Read the model definition and answer for the solid it produces. Units are mm, in the model's axes. A direction names the side the tool comes from. Give positions to 0.01 mm unless a question says otherwise; leave off trailing zeros. Write each loop counter-clockwise with the first axis right and the second up, starting at its lowest first coordinate (ties: lowest second). Pieces come first, ordered by that corner, then holes. Notation, with made-up numbers: M 53.25,58 L 80.25,58 A6 cw 80.25,68 Z; hole C 48,67 d7. An arc over 180 degrees is marked long. Put each result on its own line as item: value.
Autodesk Inventor part; units mm, degrees
ref_plane "YZ Plane" through (0, 0, 0) normal (1, 0, 0) x (0, 1, 0)
ref_plane "XZ Plane" through (0, 0, 0) normal (0, 1, 0) x (-1, 0, 0)
ref_plane "XY Plane" through (0, 0, 0) normal (0, 0, 1) x (1, 0, 0)
sketch "Sketch1" plane through (0, 0, 0) normal (0, 1, 0) x (-1, 0, 0)
  line L0 (0, 0) -> (-25, 0)
  line L1 (-25, 0) -> (-25, 25)
  line L2 (-25, 25) -> (0, 25)
  line L3 (0, 25) -> (0, 0)
  circle A0 centre (-4.5, 4.5) radius 4
  circle A1 centre (-4.5, 20.5) radius 4
  circle A2 centre (-20.5, 20.5) radius 4
  circle A3 centre (-20.5, 4.5) radius 4
  dimension "d0" = 25
  dimension "d1" = 25
  dimension "d2" = 8
  dimension "d3" = 8
  dimension "d4" = 8
  dimension "d5" = 8
extrude "Extrusion1" add sketch "Sketch1" along normal blind 5
sketch "Sketch2" plane through (0, 5, 0) normal (0, 1, 0) x (1, 0, 0)
  line L0 (0, 0) -> (0, -25)
  line L1 (25, -25) -> (25, 0)
  line L2 (0, -25) -> (25, -25)
  line L3 (25, -25) -> (25, 0)
  line L4 (25, 0) -> (0, 0)
  line L5 (0, 0) -> (0, -25)
extrude "Extrusion2" add sketch "Sketch2" along normal blind 5
sketch "Sketch4" plane through (0, 0, 0) normal (0, -1, 0) x (1, 0, 0)
  line L0 (9.5, 3) -> (15.5, 3)
  line L1 (15.5, 3) -> (15.5, 6)
  line L2 (15.5, 6) -> (9.5, 6)
  line L3 (9.5, 6) -> (9.5, 3)
  line L4 (9.5, 22) -> (15.5, 22)
  line L5 (15.5, 22) -> (15.5, 19)
  line L6 (15.5, 19) -> (9.5, 19)
  line L7 (9.5, 19) -> (9.5, 22)
  point P0 (0, 0)
  dimension "d12" = 6
  dimension "d13" = 3
  dimension "d14" = 6
  dimension "d15" = 3
extrude "Extrusion3" add sketch "Sketch4" along normal blind 5
sketch "Sketch5" plane through (0, -5, 0) normal (0, -1, 0) x (1, 0, 0)
  line L0 (15.5, 3) -> (15.5, 6)
  line L1 (9.5, 6) -> (9.5, 3)
  line L2 (15.5, 4) -> (9.5, 4)
  line L3 (9.5, 4) -> (9.5, 5)
  line L4 (9.5, 5) -> (15.5, 5)
  line L5 (15.5, 5) -> (15.5, 4)
  line L6 (15.5, 19) -> (15.5, 22)
  line L7 (15.5, 21) -> (9.5, 21)
  line L8 (9.5, 21) -> (9.5, 20)
  line L9 (9.5, 20) -> (15.5, 20)
  line L10 (15.5, 20) -> (15.5, 21)
  point P0 (0, 0)
  dimension "d18" = 1
  dimension "d19" = 6
  dimension "d20" = 1
extrude "Extrusion4" add sketch "Sketch5" along normal blind 4
sketch "Sketch6" plane through (0, -9, 0) normal (0, -1, 0) x (1, 0, 0)
  line L0 (15.5, 6) -> (15.5, 3)
  line L1 (9.5, 3) -> (9.5, 6)
  line L2 (15.5, 5.5) -> (9.5, 5.5)
  line L3 (9.5, 5.5) -> (9.5, 3.5)
  line L4 (9.5, 3.5) -> (15.5, 3.5)
  line L5 (15.5, 3.5) -> (15.5, 5.5)
  line L6 (15.5, 22) -> (15.5, 19)
  line L7 (15.5, 21.45) -> (9.5, 21.45)
  line L8 (9.5, 21.45) -> (9.5, 19.45)
  line L9 (9.5, 19.45) -> (15.5, 19.45)
  line L10 (15.5, 19.45) -> (15.5, 21.45)
  point P0 (0, 0)
  dimension "d23" = 2
  dimension "d24" = 6
  dimension "d25" = 2
extrude "Extrusion5" add sketch "Sketch6" along normal blind 1
sketch "Sketch7" plane through (15.5, -9, 19.45) normal (0, 0, -1) x (-1, 0, 0)
  line L0 (0, 0) -> (0, -1)
  line L1 (6, 4) -> (6, 0)
  line L2 (0, -1) -> (6, -1)
  line L3 (6, -1) -> (6, 3.5)
  line L4 (6, 3.5) -> (0, 3.5)
  line L5 (0, 3.5) -> (0, -1)
  point P0 (15.5, 9)
  dimension "d28" = 4.5
extrude "Extrusion6" add sketch "Sketch7" along normal blind 1
sketch "Sketch8" plane through (9.5, -9, 21.45) normal (0, 0, 1) x (1, 0, 0)
  line L0 (6, 0) -> (6, -1)
  line L1 (0, 4) -> (0, 0)
  line L2 (6, -1) -> (0, -1)
  line L3 (0, -1) -> (0, 3.5)
  line L4 (0, 3.5) -> (6, 3.5)
  line L5 (6, 3.5) -> (6, -1)
  point P0 (-9.5, 9)
  dimension "d31" = 4.5
extrude "Extrusion7" add sketch "Sketch8" along normal blind 1
sketch "Sketch9" plane through (9.5, -9, 5.5) normal (0, 0, 1) x (1, 0, 0)
  line L0 (6, -1) -> (0, -1)
  line L1 (0, 4) -> (0, 0)
  line L2 (6, -1) -> (0, -1)
  line L3 (0, -1) -> (0, 3.5)
  line L4 (0, 3.5) -> (6, 3.5)
  line L5 (6, 3.5) -> (6, -1)
  point P0 (-9.5, 9)
  dimension "d34" = 4.5
extrude "Extrusion8" add sketch "Sketch9" along normal blind 1
sketch "Sketch10" plane through (15.5, -9, 3.5) normal (0, 0, -1) x (-1, 0, 0)
  line L0 (6, 0) -> (6, -1)
  line L1 (0, 3.5) -> (6, 3.5)
  line L2 (6, -1) -> (0, -1)
  line L3 (0, -1) -> (0, 3.5)
  line L4 (0, 3.5) -> (6, 3.5)
  line L5 (6, 3.5) -> (6, -1)
  point P0 (15.5, 9)
  dimension "d37" = 4.5
extrude "Extrusion9" add sketch "Sketch10" along normal blind 1
chamfer "Chamfer1" distance 1.5 angle 45 1 edges at (12.5, -10, 2.5)
chamfer "Chamfer2" distance 1.5 angle 45 1 edges at (12.5, -10, 6.5)
fillet "Fillet1" radius 2 2 edges at (12.5, -8.5, 2.5) (12.5, -8.5, 6.5)
fillet "Fillet2" radius 1 2 edges at (12.5, -10, 5) (12.5, -10, 4)
chamfer "Chamfer3" distance 1.5 angle 45 2 edges at (12.5, -10, 18.45) (12.5, -10, 22.45)
fillet "Fillet3" radius 1 2 edges at (12.5, -10, 20.95) (12.5, -10, 19.95)
fillet "Fillet4" radius 2 2 edges at (12.5, -8.5, 22.45) (12.5, -8.5, 18.45)
sketch "Sketch11" plane through (0, 10, 0) normal (0, 1, 0) x (1, 0, 0)
  circle A0 centre (12.5, -12.5) radius 0.75
  point P0 (0, 0)
  dimension "d53" = 1.5
hole "Hole1" at (12.5, 10, 12.5) direction (0, -1, 0) diameter 1.5 depth 10
properties part number "SiPM outer housing"
(1) Section B-B on y = -4.25 is taken. Determine the outline of the cut face in (x, z).
Result:
outline: M 9.5,3 L 15.5,3 L 15.5,6 L 9.5,6 Z; M 9.5,19 L 15.5,19 L 15.5,22 L 9.5,22 Z
(2) Given pin 1 Ø1.5 at (x, y) = (13, -1.5) entering from -Z; pin 2 Ø1.1 at (x, y) = (13.5, -7) entering from +Z; pin 3 Ø6.5 at (x, z) = (4.5, 4.5) entering from -Y, each flat-ended and moving along its own axis, determine where each tip first touches the part or whether it passes through.
Result:
pin 1: stops at z = 3
pin 2: stops at z = 22.45
pin 3: stops at y = 5
(3) Straight lines are drawn through the part: line 1 along Z through (x, y) = (20.5, 1.8); line 2 along X through (y, z) = (6, 12.5). For each, find the intervals that lie inside material, in ascending order. Write a range as from..to.
Result:
line 1: z = 0..0.5, 8.5..16.5, 24.5..25
line 2: x = 0..11.75, 13.25..25
(4) Section D-D on x = 20.5 is taken. Determine the outline of the cut face in (y, z), and give its area (3 significant figures).
Result:
outline: M 0,0 L 10,0 L 10,25 L 0,25 L 0,24.5 L 5,24.5 L 5,16.5 L 0,16.5 L 0,8.5 L 5,8.5 L 5,0.5 L 0,0.5 Z
area: 170 mm²
(5) Section A-A on z = 12.5 is taken. Determine the outline of the cut face in (x, y), and give its area (3 significant figures).
Result:
outline: M 0,0 L 11.75,0 L 11.75,10 L 0,10 Z; M 13.25,0 L 25,0 L 25,10 L 13.25,10 Z
area: 235 mm²
(6) For a pull along X with two mould halves and no side action, classify faces 1 (the face through (25, 5, 12)), 2 (the face through (5.367, 2.465, 8.405)), 3 (the face through (20, 5, 20)), 4 (the face through (12, -5.5, 19)) as +X half, -X half, draft (parallel to the pull), parting line (faces both ways), or undercut.
Result:
face 1: +X half
face 2: undercut
face 3: undercut
face 4: draft
(7) Which of the six approach directions +Z, -Z, +X, -X, +Y, -Y give full straight-line access (tool end or side, diameter ignored) to faces 5 (the face through (13, -2, 19)), 6 (the face through (23.45, 2.46, 17.8)), 7 (the face through (12.5, -5, 3.5))?
Result:
face 5: +X, -X
face 6: -Y
face 7: -Z, +X, -X
(8) Section C-C on y = 4.5 is taken. Determine the outline of the cut face in (x, z).
Result:
outline: M 0,0 L 25,0 L 25,25 L 0,25 Z; hole C 4.5,4.5 d8; hole C 4.5,20.5 d8; hole C 12.5,12.5 d1.5; hole C 20.5,4.5 d8; hole C 20.5,20.5 d8
